```python
from build123d import *

# Parameters (mm, degrees)
SKETCH1_W               = 8
SKETCH1_H               = 8
BOSS_EXTRUDE1_DEPTH     = 40
SKETCH2_R               = 2.75
CUT_EXTRUDE1_DEPTH      = 18
SKETCH4_R               = 0.75
CUT_EXTRUDE2_DEPTH      = 19
SKETCH2_5_R             = 4
CUT_EXTRUDE3_DEPTH      = 30
CUT_EXTRUDE3_DEPTH_BACK = 2


with BuildPart() as part:
    # Sketch1 → Boss-Extrude1 (new body)
    with BuildSketch(Plane.XY):
        Polygon((-7, 7), (-7, -7), (-7, -9), (7, -9), (7, -7), (7, 7), align=None)
        Rectangle(SKETCH1_W, SKETCH1_H, mode=Mode.SUBTRACT)
    extrude(amount=BOSS_EXTRUDE1_DEPTH)

    # Sketch2 → Cut-Extrude1 (cut)
    with BuildSketch(Plane(origin=(0, -4, 0), x_dir=(1, 0, 0), z_dir=(0, 1, 0))):
        with Locations((0, -20)):
            Circle(SKETCH2_R)
    extrude(amount=-CUT_EXTRUDE1_DEPTH, mode=Mode.SUBTRACT)

    # Sketch4 → Cut-Extrude2 (cut)
    with BuildSketch(Plane(origin=(0, 7, 0), x_dir=(1, 0, 0), z_dir=(0, 1, 0))):
        with Locations((0, -3)):
            Circle(SKETCH4_R)
        with Locations((0, -37)):
            Circle(SKETCH4_R)
    extrude(amount=-CUT_EXTRUDE2_DEPTH, mode=Mode.SUBTRACT)

    # Sketch2_5 → Cut-Extrude3 (cut, two sides)
    with BuildSketch(Plane(origin=(0, -4, 0), x_dir=(1, 0, 0), z_dir=(0, 1, 0))) as cut_extrude3_sk:
        with Locations((0, -20)):
            Circle(SKETCH2_5_R)
    extrude(amount=CUT_EXTRUDE3_DEPTH, mode=Mode.SUBTRACT)
    extrude(cut_extrude3_sk.sketch, amount=-CUT_EXTRUDE3_DEPTH_BACK, mode=Mode.SUBTRACT)


solid = part.part
```
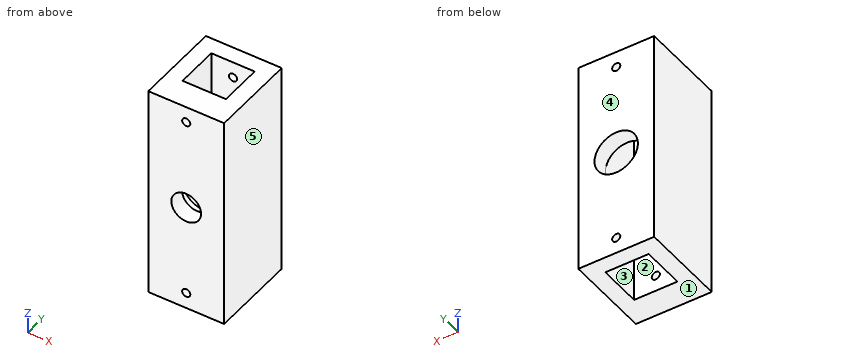
The listing builds one solid part. Answer for the finished solid, in the listing's coordinates (mm). Face numbers are marked on the shaded views. A direction names the side the tool comes from. Give positions to 0.01 mm unless a question says otherwise; leave off trailing zeros. Write each loop counter-clockwise with the first axis right and the second up, starting at its lowest first coordinate (ties: lowest second). Pieces come first, ordered by that corner, then holes. Notation, with made-up numbers: M -30,-2.75 L -17,-2.75 A27 cw -17,25.25 Z; hole C -25,45.25 d6. An arc over 180 degrees is marked long. Write each question's results on one line, items separated by ' | '.
Q1. A tool of negligible diameter and unlimited length cuts with its end or side. For the marked faces 1 and 2, from which of +Z, -Z, +X, -X, +Y, -Y can it reach the whole face along a straight path? Write none if from no direction.
Output values:
face 1: -Z, +X, -X, +Y, -Y | face 2: +Z, -Z
Q2. Section C-C, the plane x = 1.25 is taken. Write down the section's boundary in (y, z).
Output values:
outline: M -9,0 L -4,0 L -4,16.2 L -6,16.2 L -6,17.55 L -9,17.55 Z; M -9,22.45 L -6,22.45 L -6,23.8 L -4,23.8 L -4,40 L -9,40 Z; M 4,0 L 7,0 L 7,16.2 L 4,16.2 Z; M 4,23.8 L 7,23.8 L 7,40 L 4,40 Z
Q3. Section A-A, the plane z = 37 is taken. Write down the section's boundary in (x, y), then the cut area to 3 significant figures.
Output values:
outline: M -7,-9 L -0.75,-9 L -0.75,-4 L -4,-4 L -4,4 L -0.75,4 L -0.75,7 L -7,7 Z; M 0.75,-9 L 7,-9 L 7,7 L 0.75,7 L 0.75,4 L 4,4 L 4,-4 L 0.75,-4 Z | area: 148 mm2
Q4. Section D-D, the plane z = 30 is taken. Write down the section's boundary in (x, y), then the cut area to 3 significant figures.
Output values:
outline: M -7,-9 L 7,-9 L 7,7 L -7,7 Z; hole M -4,-4 L 4,-4 L 4,4 L -4,4 Z | area: 160 mm2
Q5. Section B-B, the plane y = -2.5 is taken. Write down the section's boundary in (x, z).
Output values:
outline: M -7,0 L -4,0 L -4,40 L -7,40 Z; M 4,0 L 7,0 L 7,40 L 4,40 Z
Q6. Consider L1, parallel to Z at x = 0, y = -7.7; L2, parallel to Z at x = 0, y = 5.75; L3, parallel to Y at x = 1, z = 32.5. Determine where each line is inside the solid, lowest interval first. Write a range as from..to.
Output values:
L1: 0..2.25, 3.75..17.25, 22.75..36.25, 37.75..40 | L2: 0..2.25, 3.75..16, 24..36.25, 37.75..40 | L3: -9..-4, 4..7
Q7. For a pull along X with two mould halves and no side action, classify the marked faces 3, 4 and 5 as released by +X, released by -X, zero draft, split by the parting line, or undercut.
Output values:
face 3: undercut | face 4: zero draft | face 5: released by +X
